from build123d import *

# Parameters (mm, degrees)
SKETCH1_W                       = 65
SKETCH1_H                       = 16
SKETCH1_W_2                     = 31
SKETCH1_H_2                     = 32
BOSS_EXTRUDE1_DEPTH             = 105
SKETCH2_R                       = 7
CUT_EXTRUDE1_DEPTH              = 105
BOSS_EXTRUDE2_REACH             = 62.226
SKETCH8_R                       = 15
SKETCH8_R_2                     = 10.5
BOSS_EXTRUDE2_DIRECTION_2_REACH = 55.245
SKETCH8_2_R                     = 10.5
CUT_EXTRUDE2_DEPTH              = 61.225525817
CUT_EXTRUDE2_DEPTH_BACK         = 54.244882879
FILLET2_R                       = 5


with BuildPart() as part:
    # Sketch1 → Boss-Extrude1 (new body)
    with BuildSketch(Plane(origin=(0, 0, 0), x_dir=(1, 0, 0), z_dir=(0, 1, 0))):
        Rectangle(SKETCH1_W, SKETCH1_H)
        with Locations((0, -8)):
            Rectangle(SKETCH1_W_2, SKETCH1_H_2)
    extrude(amount=BOSS_EXTRUDE1_DEPTH)

    # Sketch2 → Cut-Extrude1 (cut)
    with BuildSketch(Plane(origin=(0, 0, -8), x_dir=(-1, 0, 0), z_dir=(0, 0, -1))):
        with Locations((0, 90)):
            Circle(SKETCH2_R)
        with Locations((0, 15)):
            Circle(SKETCH2_R)
    extrude(amount=-CUT_EXTRUDE1_DEPTH, mode=Mode.SUBTRACT)

    # Boss-Extrude2: up to this face of the body (flat: up to its plane)
    boss_extrude2_end = Plane(part.part.faces().sort_by_distance((-32.5, 52.5, 0))[0])
    # Sketch8 → Boss-Extrude2 (add, up to the picked face)
    with BuildSketch(Plane(origin=(27.526035262, 19.273937388, 0), x_dir=(0, 0, 1), z_dir=(-0.819152044, -0.573576436, 0)), mode=Mode.PRIVATE) as boss_extrude2_sk1:
        with Locations((-8, 43.005482325)):
            Circle(SKETCH8_R)
        with Locations((-8, 43.005482325)):
            Circle(SKETCH8_R_2, mode=Mode.SUBTRACT)
    boss_extrude2_tool1 = split(extrude(boss_extrude2_sk1.sketch, amount=BOSS_EXTRUDE2_REACH, mode=Mode.PRIVATE), bisect_by=boss_extrude2_end, keep=Keep.BOTH, mode=Mode.PRIVATE)
    add(boss_extrude2_tool1.solids().sort_by_distance((2.859104, 54.501966, -22.575736))[0])

    # Boss-Extrude2 direction 2: up to this face of the body (flat: up to its plane)
    boss_extrude2_direction_2_end = Plane(part.part.faces().sort_by_distance((32.5, 52.5, 0))[0])
    # Sketch8 → Boss-Extrude2 direction 2 (add, up to the picked face)
    with BuildSketch(Plane(origin=(27.526035262, 19.273937388, 0), x_dir=(0, 0, 1), z_dir=(-0.819152044, -0.573576436, 0)), mode=Mode.PRIVATE) as boss_extrude2_direction_2_sk1:
        with Locations((-8, 43.005482325)):
            Circle(SKETCH8_R)
        with Locations((-8, 43.005482325)):
            Circle(SKETCH8_R_2, mode=Mode.SUBTRACT)
    boss_extrude2_direction_2_tool1 = split(extrude(boss_extrude2_direction_2_sk1.sketch, amount=-BOSS_EXTRUDE2_DIRECTION_2_REACH, mode=Mode.PRIVATE), bisect_by=boss_extrude2_direction_2_end, keep=Keep.BOTH, mode=Mode.PRIVATE)
    add(boss_extrude2_direction_2_tool1.solids().sort_by_distance((2.859104, 54.501966, -22.575736))[0])

    # Sketch8<2> → Cut-Extrude2 (cut, two sides)
    with BuildSketch(Plane(origin=(27.526035262, 19.273937388, 0), x_dir=(0, 0, 1), z_dir=(-0.819152044, -0.573576436, 0))) as cut_extrude2_sk:
        with Locations((-8, 43.005482325)):
            Circle(SKETCH8_2_R)
    extrude(amount=CUT_EXTRUDE2_DEPTH, mode=Mode.SUBTRACT)
    extrude(cut_extrude2_sk.sketch, amount=-CUT_EXTRUDE2_DEPTH_BACK, mode=Mode.SUBTRACT)

    # Fillet2
    fillet2_edges = [part.edges().sort_by_distance(p)[0] for p in [
        (0, 70.811618831, -8),
        (0, 34.188381169, -8),
    ]]
    fillet(fillet2_edges, radius=FILLET2_R)


solid = part.part
Verification items for the finished model (mm, model axes). A direction names the side the tool comes from. Give positions to 0.01 mm unless a question says otherwise; leave off trailing zeros. Write each loop counter-clockwise with the first axis right and the second up, starting at its lowest first coordinate (ties: lowest second). Pieces come first, ordered by that corner, then holes. Notation, with made-up numbers: M -37.5,64 L -8.5,64 A25 cw -8.5,82 Z; hole C 35.5,57 d5. An arc over 180 degrees is marked long. Put each result on its own line as item: value. Start each with the question number.
1. Section check A-A (z = 1). Record the cut outline in (x, y), and give its area (3 significant figures).
2. Draft check along X on faces 1 (the face through (24, 52, 8)), 2 (the face through (32.5, 52, 0)), 3 (the face through (1.517, 8.166, 7.776)). Enter one of: +X half, -X half, draft (parallel to the pull), parting line (faces both ways), or undercut.
3. Go/stop test with flat-tipped pins: pin 1 Ø2 at (y, z) = (18, -8.5) entering from -X; pin 2 Ø8.5 at (x, y) = (-22.5, 37.5) entering from +Z; pin 3 Ø3 at (x, y) = (-4.5, 18.5) entering from -Z. Record where each tip stops, or that it passes through.
4. Section check C-C (x = 5.5). Give the number of separate pieces and of enclosed holes in the cut face, and give its area (3 significant figures).
5. Scan lines: line 1 along Y through (x, z) = (0, 17); line 2 along Z through (x, y) = (9, 100); line 3 along Y through (x, z) = (-15, -2.5). Record each from-to range of solid material in increasing order. Write a range as [from, to].
6. Set-up check for faces 4 (the face through (15.5, 52, 16)), 5 (the face through (-7, 85, -8)), 6 (the face through (8, 20, -8)), 7 (the face through (-24, 52, 8)), 8 (the face through (0, 52, 24)): record each of +Z, -Z, +X, -X, +Y, -Y from which the full face is reachable in a straight line by a thin tool's end or side.
7. Section check B-B (z = -10). Record the cut outline in (x, y), and give its area (3 significant figures).
Answer list:
1. outline: M -32.5,0 L 32.5,0 L 32.5,68.65 L -32.5,23.14 Z; M -32.5,36.35 L 32.5,81.86 L 32.5,105 L -32.5,105 Z; hole C 0,15 d14; hole C 0,90 d14
1. area: 5,660 mm2
2. face 1: draft
2. face 2: +X half
2. face 3: undercut
3. pin 1: x = -32.42
3. pin 2: z = 8
3. pin 3: z = -8
4. separate pieces: 3
4. enclosed holes: 1
4. area: 2,820 mm2
5. line 1: [0, 8], [22, 83], [97, 105]
5. line 2: [-8, 24]
5. line 3: [0, 31.08], [52.92, 105]
6. face 4: +Z, +X, +Y, -Y
6. face 5: -Z, -X, +Y
6. face 6: -Z, +X, -Y
6. face 7: +Z, -X, +Y, -Y
6. face 8: +Z, +X, -X, +Y, -Y
7. outline: M -32.5,10.99 L 32.5,56.5 L 32.5,62.67 L -32.5,17.16 Z; M -32.5,42.33 L 32.5,87.84 L 32.5,94.01 L -32.5,48.5 Z
7. area: 803 mm2
